Could you check a few things on this model? Use its own coordinates, in mm. Face numbers are marked on the shaded views. A direction names the side the tool comes from. Give positions to 0.01 mm unless a question says otherwise; leave off trailing zeros. Loops run counter-clockwise (first coordinate to the right, second up) from the corner with the lowest first, then second, coordinate; pieces in that order, holes last. Notation, with made-up numbers: M 34,-22.5 L 48,-22.5 A8 cw 48,-11.5 Z; hole C 32,-25 d10. An arc over 180 degrees is marked long. Use a Markdown table: item, result. Add a question column.
1) Suppose I cut it at A-A on y = 1.5. List the corners of the cut face in (x, z) for me, and give its area (3 significant figures).
2) Which directions (+Z, -Z, +X, -X, +Y, -Y) give clear straight access to the entire face, cutting with the end or side of a thin tool? Please do the marked faces 5, 6 and 7.
3) Will these pins go through, and if not, where does the flat tip stop? pin 1 Ø3 at (x, z) = (4.5, -3) entering from -Y; pin 2 Ø1.9 at (y, z) = (-1.5, -8.5) entering from -X; pin 3 Ø4 at (x, z) = (-5, 1) entering from -Y.
4) If I drill on line 1 along Y through (x, z) = (-6.5, 0.5); line 2 along Y through (x, z) = (4.5, -3.25); line 3 along Z through (x, y) = (0, -1.25), over which ranges is the centre line in solid material (lowest first)? Write a range as [from, to].
5) We'd pull the mould along Z, two halves only. Please class the marked faces 1, 2, 3 and 4: +Z half, -Z half, draft (parallel to the pull), parting line (faces both ways), or undercut.
Autodesk Inventor part; units mm, degrees
ref_plane "YZ Plane" through (0, 0, 0) normal (1, 0, 0) x (0, 1, 0)
ref_plane "XZ Plane" through (0, 0, 0) normal (0, 1, 0) x (-1, 0, 0)
ref_plane "XY Plane" through (0, 0, 0) normal (0, 0, 1) x (1, 0, 0)
sketch "Sketch1" plane through (0, 0, 0) normal (0, 0, 1) x (1, 0, 0)
  line L0 (-3.8177, -2.5414) -> (-3.8177, 2.9086)
  line L1 (-3.8177, 2.9086) -> (8.4464, 2.9086)
  line L2 (8.4323, 2.6586) -> (8.4323, -2.5414)
  line L3 (8.4323, -2.5414) -> (-3.8177, -2.5414)
  line L4 (-3.8177, 8.4062) -> (-3.8177, -10.1402)
  line L5 (8.4323, 2.6586) -> (8.5573, 2.9086)
  line L6 (8.5573, 2.9086) -> (8.4464, 2.9086)
  point P0 (0, 0)
  dimension "d1" = 24.5
  dimension "d2" = 5.45
  dimension "d29" = 0.25
  dimension "d30" = 24.75
revolve "Revolution1" add sketch "Sketch1" angle 360 about axis through (-3.8177, 8.4062, 0) along (0, -1, 0)
sketch "Sketch2" plane through (-3.8177, -2.5414, 0) normal (0, -1, 0) x (1, 0, 0)
  circle A0 centre (0, 0) radius 12.75 construction
  circle A1 centre (0, 0) radius 12.25
  line L0 (0, 12.75) -> (0, -12.75) construction
  line L1 (-5.3884, -11.5554) -> (5.3884, 11.5554) construction
  line L2 (-5.3884, 11.5554) -> (5.3884, -11.5554) construction
  circle A2 centre (-5.3884, -11.5554) radius 1.1
  circle A3 centre (5.3884, -11.5554) radius 1.1
  circle A4 centre (0, 12.75) radius 1.1
  point P0 (3.8177, 0)
  dimension "d4" = 25.5
  dimension "d5" = 25
  dimension "d6" = 25
  dimension "d7" = 2.2
extrude "Extrusion1" cut sketch "Sketch2" against normal blind 4.75 contours A4 A1 | A1 A4 | A3 A1 | A1 A3 | A2 A1 | A1 A2
sketch "Sketch3" plane through (-3.8177, -2.5414, 0) normal (0, -1, 0) x (1, 0, 0)
  line L0 (-12.375, -7.5) -> (9.1567, -7.5)
  line L1 (9.1567, 7.5) -> (-12.375, 7.5)
  circle A0 centre (0, 0) radius 9.9629 construction
  line L2 (-12.375, 7.5) -> (-12.375, -7.5)
  line L3 (9.1567, -7.5) -> (9.1567, 7.5)
  circle A1 centre (0, 0) radius 12.375
  point P0 (-9.8433, -7.5)
  dimension "d11" = 15
  dimension "d92" = 7.5
  dimension "d94" = 19
extrude "Extrusion2" cut sketch "Sketch3" against normal up to surface (4.75 mm away) contours L2 A1 L0 | A1 L1 L3 L0 | L2 L1 A1 picked at (1.9795, 0)
sketch "Sketch5" plane through (-13.5034, 2.2086, 7.5) normal (0, -1, 0) x (1, 0, 0)
  line L0 (14.6857, -2.5) -> (4.6857, -2.5)
  line L1 (4.6857, -2.5) -> (4.6857, -12.5)
  line L2 (4.6857, -12.5) -> (14.6857, -12.5)
  line L3 (14.6857, -12.5) -> (14.6857, -2.5)
  line L4 (14.6857, -2.5) -> (4.6857, -12.5) construction
  line L5 (4.6857, -2.5) -> (14.6857, -12.5) construction
  line L6 (-1.8929, -11.5) -> (-2.0018, -11.5)
  arc A0 (0, 0) -> (0, -15) centre (9.6857, -7.5) ccw
  arc A1 (0.7907, -0.6122) -> (0.7907, -14.3878) centre (9.6857, -7.5) ccw
  line L7 (4.6857, -11.25) -> (-0.9209, -11.25)
  line L8 (-1.223, -10.25) -> (4.6857, -10.25)
  point P0 (4.6857, -11.5)
  dimension "d95" = 10
  dimension "d99" = 1
  dimension "d100" = 1
  dimension "d101" = 1.25
extrude "Extrusion3" cut sketch "Sketch5" against normal blind 0.25
sketch "Sketch7" plane through (-3.8177, 2.9086, 0) normal (0, 1, 0) x (1, 0, 0)
  arc A0 (12.3346, 0.9992) -> (12.3346, -0.9992) centre (12.375, 0) ccw
  circle A1 centre (0, 0) radius 12.375
  arc A2 (-12.3346, -0.9992) -> (-12.3346, 0.9992) centre (-12.375, 0) ccw
  line L0 (-12.375, 0) -> (12.375, 0) construction
  dimension "d34" = 2
extrude "Extrusion5" [suppressed]
ref_plane "Work Plane1" through (-13.5034, 0.0586, -7.5) normal (1, 0, 0) x (0, 1, 0)
ref_plane "Work Plane3" through (-16.0677, 0.0586, 0) normal (-1, 0, 0) x (0, -1, 0)
ref_plane "Work Plane2" through (5.339, -2.5414, 0) normal (0, 0, -1) x (-1, 0, 0)
sketch "Sketch10" plane through (-13.5034, 0.0586, -7.5) normal (1, 0, 0) x (0, 1, 0)
  line L0 (-0.8679, 15) -> (-0.8679, 17)
  line L1 (-0.8679, 17) -> (-2.6, 16)
  line L2 (2.15, 15) -> (-2.6, 15)
  line L3 (-2.6, 19.7124) -> (-2.6, 15)
  line L4 (-2.6, 0) -> (2.15, 0)
  line L5 (-2.6, 0) -> (-2.6, -3.1626)
  point P0 (-0.0586, 7.5)
  dimension "d69" = 60
  dimension "d70" = 1
  dimension "d71" = 2
extrude "Extrusion8" cut sketch "Sketch10" along normal blind 16
mirror "Mirror1" about plane through (5.339, -2.5414, 0) normal (0, 0, -1) of "Extrusion8"
chamfer "Chamfer2" distance 0.25 angle 45 3 edges at (-8.7412, -2.5414, -10.5585) (1.1058, -2.5414, -10.5585) (-3.8177, -2.5414, 11.65)
sketch "Sketch11" plane through (5.339, -2.5414, -7.5) normal (0, -1, 0) x (1, 0, 0)
  arc A0 (-10.3843, 19.6883) -> (-7.9291, 19.6883) centre (-9.1567, 20.25) ccw
  arc A1 (-10.3843, 19.6883) -> (-17.9778, 16) centre (-9.1567, 7.5) ccw
  line L0 (-17.9778, 16) -> (-2.8424, 16)
  line L1 (-2.8424, 16) -> (-2.8424, 15)
  line L2 (-2.8424, 15) -> (0, 15)
  line L3 (0, 15) -> (0, 0)
  line L4 (0, 0) -> (-2.8424, 0)
  line L5 (-2.8424, 0) -> (-2.8424, -1)
  line L6 (-2.8424, -1) -> (-17.9778, -1)
  arc A2 (-17.9778, -1) -> (-15.4203, -3.0276) centre (-9.1567, 7.5) ccw
  arc A3 (-13.1951, -4.0652) -> (-15.4203, -3.0276) centre (-14.5451, -4.0554) ccw
  arc A4 (-13.1951, -4.0652) -> (-5.1183, -4.0652) centre (-9.1567, 7.5) ccw
  arc A5 (-2.8931, -3.0276) -> (-5.1183, -4.0652) centre (-3.7683, -4.0554) ccw
  arc A6 (-2.8931, -3.0276) -> (-7.9291, 19.6883) centre (-9.1567, 7.5) ccw
  line L7 (0, 0.1) -> (0.6056, 0.1)
  line L8 (0, 14.9) -> (0.6056, 14.9)
  line L9 (-18.8424, 0) -> (-2.8424, 0)
  dimension "d82" = 0.1
  dimension "d83" = 0.1
extrude "Extrusion9" add sketch "Sketch11" along normal blind 1.5 contours A6 L7 L3 L8
chamfer "Chamfer3" distance 0.5 angle 45 2 edges at (5.339, -0.1664, 7.5) (5.339, -0.1664, -7.5)
sketch "Sketch12" plane through (5.339, -4.0414, -7.5) normal (0, -1, 0) x (1, 0, 0)
  circle A0 centre (1.8433, 7.5) radius 0.4
  circle A1 centre (-9.1567, 7.5) radius 12.25 construction
  arc A2 (-13.1951, -4.0652) -> (-5.1183, -4.0652) centre (-9.1567, 7.5) ccw
  dimension "d87" = 11
  dimension "d88" = 0.8
extrude "Extrusion10" add sketch "Sketch12" along normal blind 0.3
fillet "Fillet1" radius 0.25 2 edges at (6.7823, -4.0414, 0) (6.7823, -4.3414, 0)
equation "\"d92\" = 0.5 * d11"
properties part number "bottom1_2_bigtouch" material "Acrylic"
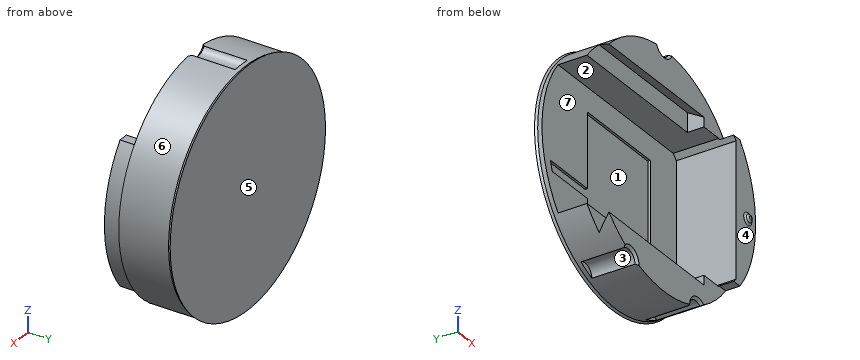
Answer block:
| question | item | result |
|---|---|---|
| 1 | outline | M -13.5,-7.5 A12.25 ccw -9.85,-10.66 A1.1 cw -8.11,-11.47 A12.25 ccw 0.47,-11.47 A1.1 cw 2.21,-10.66 A12.25 ccw -2.86,12.21 A1.1 cw -4.78,12.21 A12.25 ccw -13.5,7.5 L 4.84,7.5 L 5.34,7 L 5.34,-7 L 4.84,-7.5 Z |
| 1 | area | 160 mm^2 |
| 2 | face 5 | +Z, -Z, +X, -X, +Y |
| 2 | face 6 | -Y |
| 2 | face 7 | -X, -Y |
| 3 | pin 1 | stops at y = -4.04 |
| 3 | pin 2 | stops at x = -13.22 |
| 3 | pin 3 | stops at y = 2.46 |
| 4 | line 1 | y = [2.46, 2.91] |
| 4 | line 2 | y = [2.21, 2.91] |
| 4 | line 3 | z = [-11.64, -9.25], [9.25, 11.64] |
| 5 | face 1 | undercut |
| 5 | face 2 | undercut |
| 5 | face 3 | -Z half |
| 5 | face 4 | draft |
